Read the model definition and answer for the solid it produces. Units are mm, in the model's axes. Face numbers are marked on the shaded views. Coordinates: 2 decimals unless noted, no trailing zeros. Loops run counter-clockwise (first coordinate to the right, second up) from the corner with the lowest first, then second, coordinate; pieces in that order, holes last. Notation, with made-up numbers: (48.5, -11.5) -> (87.5, -11.5) arc R15 cw to (87.5, 12.5) -> close; hole circle Ø8 at (-3.75, 40.5). An arc over 180 degrees is marked (long way). Answer as a JSON object with one key per item and string values. Group by question number.
1) Flat-ended cylindrical pins translate along their axes: P1, Ø4, axis at x = -36, z = 31.5, coming from the -Y side; P2, Ø1.5, axis at x = 42.5, z = 0, coming from the -Y side. Find the tip coordinate at first contact, or state that the pin passes through.
2) Determine the mould class of the marked faces 1, 2, 3 and 4 for opening direction X: released by +X, released by -X, zero draft, split by the parting line, or undercut.
3) Consider probe 1 along Z at (x, y) = (42.5, -21.05); probe 2 along Y at (x, z) = (27.5, 40.5). Determine where each line is inside the solid, lowest interval first. Write a range as [from, to].
4) Section B-B, the plane x = 20 is taken. Give the vertices of the cut face in (y, z), plus the area to 4 significant figures.
5) Section A-A, the plane z = -47.5 is taken. Give the vertices of the cut face in (x, y).
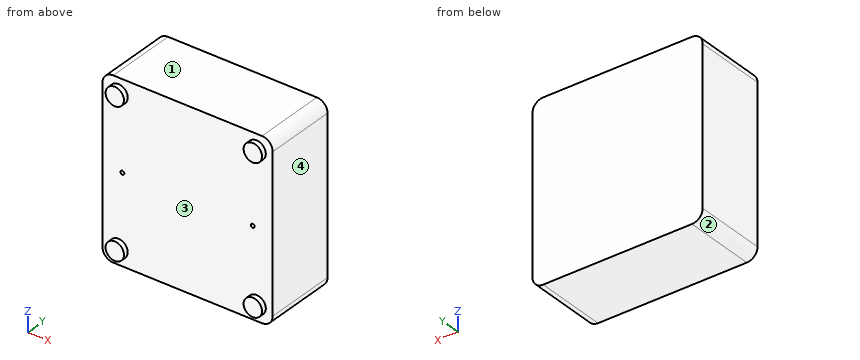
from build123d import *

# Parameters (mm, degrees)
BOSS_EXTRUDE1_DEPTH       = 23.5
SKETCH4_R                 = 6
BOSS_EXTRUDE2_DEPTH       = 3.25
M3X0_5_TAPPED_HOLE1_D     = 2.5
M3X0_5_TAPPED_HOLE1_DEPTH = 4.5
M3X0_5_TAPPED_HOLE1_TIP   = 0.751075774


with BuildPart() as part:
    # Sketch3 → Boss-Extrude1 (new, symmetric)
    with BuildSketch(Plane(origin=(0, 0, 0), x_dir=(1, 0, 0), z_dir=(0, 1, 0))):
        with BuildLine():
            Line((-48.5, 57.5), (48.5, 57.5))
            ThreePointArc((48.5, 57.5), (53.449747468, 55.449747468), (55.5, 50.5))
            Line((55.5, 50.5), (55.5, -50.5))
            ThreePointArc((55.5, -50.5), (53.449747468, -55.449747468), (48.5, -57.5))
            Line((48.5, -57.5), (-48.5, -57.5))
            ThreePointArc((-48.5, -57.5), (-53.449747468, -55.449747468), (-55.5, -50.5))
            Line((-55.5, -50.5), (-55.5, 50.5))
            ThreePointArc((-55.5, 50.5), (-53.449747468, 55.449747468), (-48.5, 57.5))
        make_face()
    extrude(amount=BOSS_EXTRUDE1_DEPTH, both=True)

    # Sketch4 → Boss-Extrude2 (add)
    with BuildSketch(Plane.XZ.offset(23.5)):
        with Locations(Location((45, 47.5, 0), (0, 0, 90))):
            Circle(SKETCH4_R)
        with Locations(Location((-45, 47.5, 0), (0, 0, 90))):
            Circle(SKETCH4_R)
        with Locations(Location((-45, -47.5, 0), (0, 0, 90))):
            Circle(SKETCH4_R)
        with Locations(Location((45, -47.5, 0), (0, 0, 90))):
            Circle(SKETCH4_R)
    extrude(amount=BOSS_EXTRUDE2_DEPTH)

    # M3x0.5 Tapped Hole1
    with Locations(Plane(origin=(0, -23.5, 0), x_dir=(-1, 0, 0), z_dir=(0, -1, 0))):
        with Locations((-42.5, 0), (42.5, 0)):
            Hole(M3X0_5_TAPPED_HOLE1_D / 2, depth=M3X0_5_TAPPED_HOLE1_DEPTH)
            with Locations((0, 0, -(M3X0_5_TAPPED_HOLE1_DEPTH + M3X0_5_TAPPED_HOLE1_TIP / 2))):  # 118° drill point
                Cone(0, M3X0_5_TAPPED_HOLE1_D / 2, M3X0_5_TAPPED_HOLE1_TIP, mode=Mode.SUBTRACT)


solid = part.part
Determined:
{
 "1": {"P1": "y = -23.5", "P2": "y = -18.7"},
 "2": {"face 1": "zero draft", "face 2": "released by -X", "face 3": "undercut", "face 4": "released by +X"},
 "3": {"probe 1": "[-57.5, -1.25], [1.25, 57.5]", "probe 2": "[-23.5, 23.5]"},
 "4": {"outline": "(-23.5, -57.5) -> (23.5, -57.5) -> (23.5, 57.5) -> (-23.5, 57.5) -> close", "area": "5,405 mm²"},
 "5": {"outline": "(-55.5, -23.5) -> (-51, -23.5) -> (-51, -26.75) -> (-39, -26.75) -> (-39, -23.5) -> (39, -23.5) -> (39, -26.75) -> (51, -26.75) -> (51, -23.5) -> (55.5, -23.5) -> (55.5, 23.5) -> (-55.5, 23.5) -> close"}
}
